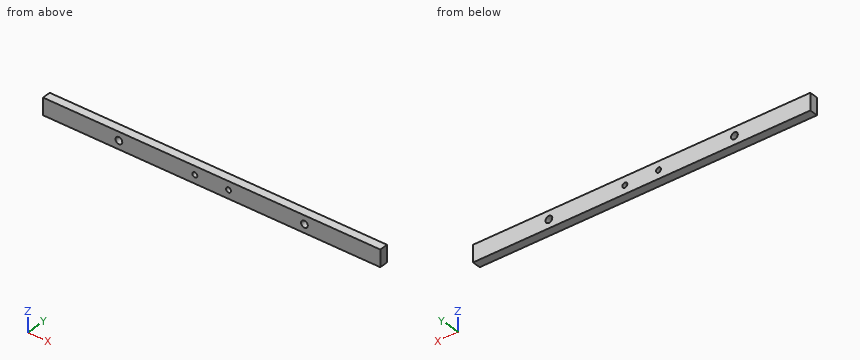
from build123d import *

# Parameters (mm, degrees)
ESQUISSE1_W             = 200
ESQUISSE1_H             = 5
BOSS_EXTRU_1_DEPTH      = 10
ESQUISSE3_R             = 2
ENL_V_MAT_EXTRU_1_DEPTH = 10
ESQUISSE3_4_R           = 2
ESQUISSE3_4_R_2         = 1.5
ENL_V_MAT_EXTRU_2_DEPTH = 10


with BuildPart() as part:
    # Esquisse1 → Boss.-Extru.1 (new body)
    with BuildSketch(Plane.XY):
        with Locations((100, -2.5)):
            Rectangle(ESQUISSE1_W, ESQUISSE1_H)
    extrude(amount=BOSS_EXTRU_1_DEPTH)

    # Esquisse3 → Enl_v. mat.-Extru.1 (cut)
    with BuildSketch(Plane.XZ.offset(5)):
        with Locations(Location((45, 5, 0), (0, 0, 270))):
            Circle(ESQUISSE3_R)
    extrude(amount=-ENL_V_MAT_EXTRU_1_DEPTH, mode=Mode.SUBTRACT)

    # Esquisse3_4 → Enl_v. mat.-Extru.2 (cut)
    with BuildSketch(Plane.XZ.offset(5)):
        with Locations(Location((45, 5, 0), (0, 0, 270))):
            Circle(ESQUISSE3_4_R)
        with Locations(Location((155, 5, 0), (0, 0, 270))):
            Circle(ESQUISSE3_4_R)
        with Locations(Location((110, 5, 0), (0, 0, 270))):
            Circle(ESQUISSE3_4_R_2)
        with Locations(Location((90, 5, 0), (0, 0, 270))):
            Circle(ESQUISSE3_4_R_2)
    extrude(amount=-ENL_V_MAT_EXTRU_2_DEPTH, mode=Mode.SUBTRACT)


solid = part.part
The listing builds one solid part. Answer for the finished solid, in the listing's coordinates (mm). Give positions to 0.01 mm unless a question says otherwise; leave off trailing zeros. Write each loop counter-clockwise with the first axis right and the second up, starting at its lowest first coordinate (ties: lowest second). Pieces come first, ordered by that corner, then holes. Notation, with made-up numbers: (37, 25.25) -> (86, 25.25) arc R19 ccw to (86, 55.25) -> close; hole circle Ø10 at (-5, -21). An arc over 180 degrees is marked (long way). One line per question, with ' | ' between items. Start each with the question number.
1. Find the intervals of material crossed by probe 1 along X at (y, z) = (-3.65, 5); probe 2 along X at (y, z) = (-4.3, 4); probe 3 along Z at (x, y) = (90, -1.05), in increasing order.
2. Section B-B (y = -3.95) is taken. Determine the outline of the cut face in (x, z), plus the area to 3 significant figures.
3. Section C-C (z = 5) is taken. Determine the outline of the cut face in (x, y), plus the area to 3 significant figures.
4. Section A-A (x = 45) is taken. Determine the outline of the cut face in (y, z).
Response values:
1) probe 1: 0 to 43, 47 to 88.5, 91.5 to 108.5, 111.5 to 153, 157 to 200 | probe 2: 0 to 43.27, 46.73 to 88.88, 91.12 to 108.88, 111.12 to 153.27, 156.73 to 200 | probe 3: 0 to 3.5, 6.5 to 10
2) outline: (0, 0) -> (200, 0) -> (200, 10) -> (0, 10) -> close; hole circle Ø4 at (45, 5); hole circle Ø3 at (90, 5); hole circle Ø3 at (110, 5); hole circle Ø4 at (155, 5) | area: 1,960 mm2
3) outline: (0, -5) -> (43, -5) -> (43, 0) -> (0, 0) -> close; (47, -5) -> (88.5, -5) -> (88.5, 0) -> (47, 0) -> close; (91.5, -5) -> (108.5, -5) -> (108.5, 0) -> (91.5, 0) -> close; (111.5, -5) -> (153, -5) -> (153, 0) -> (111.5, 0) -> close; (157, -5) -> (200, -5) -> (200, 0) -> (157, 0) -> close | area: 930 mm2
4) outline: (-5, 0) -> (0, 0) -> (0, 3) -> (-5, 3) -> close; (-5, 7) -> (0, 7) -> (0, 10) -> (-5, 10) -> close
